Model file for the job. Use its own axes, mm. A direction names the side the tool comes from. Round coordinates to 2 decimals unless told otherwise and drop trailing zeros. Order: outer loops, then holes, each group sorted by start corner. A loop starts at its lowest first (then second) coordinate and runs counter-clockwise, first axis right, second up. Notation, with made-up numbers: (-30, -6) - (-20, -6) arc R18 ccw to (-20, 19) - close; hole circle Ø8 at (-15.5, 43.25). An arc over 180 degrees is marked (long way). Use one line per item in the form item = value.
Autodesk Inventor part; units mm, degrees
ref_plane "Work Plane1" through (-10, 0, 0) normal (1, 0, 0) x (0, 1, 0)
ref_plane "XZ Plane" through (0, 0, 0) normal (0, 1, 0) x (-1, 0, 0)
ref_plane "XY Plane" through (0, 0, 0) normal (0, 0, 1) x (1, 0, 0)
sketch "Sketch1" plane through (0, 0, 0) normal (0, 0, 1) x (1, 0, 0)
  circle A0 centre (0, 0) radius 125
  dimension "d0" = 250
extrude "Extrusion1" add sketch "Sketch1" along normal blind 10
ref_plane "Work Plane1" through (-10, 0, 0) normal (1, 0, 0) x (0, 1, 0)
sketch "Sketch2" plane through (-10, 0, 0) normal (1, 0, 0) x (0, 1, 0)
  line L0 (0, 0) -> (0, 156.8689) construction
  line L1 (125, 10) -> (-125, 10)
  line L2 (0, 10) -> (-87.5, 10)
  line L3 (-87.5, 10) -> (-87.5, 67.2767)
  line L4 (0, 10) -> (66.5, 10)
  line L5 (66.5, 10) -> (66.5, 44.5)
  line L6 (66.5, 44.5) -> (80.6421, 58.6421)
  line L7 (66.5, 44.5) -> (86.5, 44.5) construction
  line L8 (80.6421, 58.6421) -> (-7.7462, 147.0305) construction
  arc A0 (80.6421, 58.6421) -> (-7.7462, 147.0305) centre (36.448, 102.8363) ccw
  line L9 (-7.7462, 147.0305) -> (-87.5, 67.2767)
  line L10 (-7.7462, 147.0305) -> (127.2538, 147.0305) construction
  circle A1 centre (36.448, 102.8363) radius 22.75
  dimension "d4" = 87.5
  dimension "d6" = 66.5
  dimension "d7" = 34.5
  dimension "d8" = 20
  dimension "d9" = 45
  dimension "d10" = 125
  dimension "d11" = 135
  dimension "d12" = 45.5
extrude "Extrusion2" add sketch "Sketch2" against normal blind 55
fillet "Fillet1" radius 100 1 edges at (-37.5, -87.5, 67.2767)
fillet "Fillet2" radius 50 1 edges at (-37.5, 66.5, 44.5)
sketch "Sketch3" plane through (-65, 0, 0) normal (-1, 0, 0) x (0, 0, 1)
  line L0 (25.8553, -87.5) -> (10, -87.5)
  line L1 (10, -87.5) -> (25.8553, -87.5)
  arc A0 (25.8553, -87.5) -> (96.566, -58.2107) centre (25.8553, 12.5) ccw
  arc A1 (25.8553, -87.5) -> (96.566, -58.2107) centre (25.8553, 12.5) ccw
  line L2 (96.566, -58.2107) -> (147.0305, -7.7462)
  line L3 (96.566, -58.2107) -> (147.0305, -7.7462)
  arc A2 (147.0305, -7.7462) -> (58.6421, 80.6421) centre (102.8363, 36.448) ccw
  arc A3 (147.0305, -7.7462) -> (58.9231, 80.9213) centre (102.8363, 36.448) ccw
  arc A4 (23.7925, 66.5) -> (58.9231, 80.9213) centre (23.7925, 116.5) ccw
  arc A5 (23.7925, 66.5) -> (58.9231, 80.9213) centre (23.7925, 116.5) ccw
  line L4 (44.5, 66.5) -> (10, 66.5)
  line L5 (23.7925, 66.5) -> (10, 66.5)
  line L6 (10, 66.5) -> (10, -87.5)
  arc A6 (139.9594, -0.6751) -> (65.9492, 73.8056) centre (102.8363, 36.448) ccw
  line L7 (139.9594, -0.6751) -> (117.7788, -23.5781)
  line L8 (0, 0) -> (182.0155, 0) construction
  line L9 (0, -125) -> (0, 125) construction
  line L10 (10, 0) -> (10, -65) construction
  line L11 (10, -65) -> (20, -65)
  arc A7 (20, -65) -> (117.7788, -23.5781) centre (20, 71.1171) ccw
  line L12 (10, 0) -> (10, 40) construction
  arc A8 (10, 40) -> (65.9492, 73.8056) centre (-32.4537, 173.4637) ccw
  dimension "d16" = 10
  dimension "d17" = 65
  dimension "d18" = 10
  dimension "d19" = 40
extrude "Extrusion3" cut sketch "Sketch3" against normal blind 19.5 contours L6 A8 A6 L7 A7 L11
sketch "Sketch4" plane through (-45.5, 0, 0) normal (-1, 0, 0) x (0, 0, 1)
  line L0 (143.3452, 39.9686) -> (60.7799, -45.2853) construction
  line L1 (139.9594, -0.6751) -> (117.7788, -23.5781) construction
  circle A0 centre (102.8363, 36.448) radius 22.75 construction
  line L2 (102.2737, 74.1744) -> (28.4952, -2.0066) construction
  line L3 (100.9974, 75.3281) -> (145.8599, 31.8805) construction
  line L4 (22.9611, 6.1258) -> (80.8137, -49.9023) construction
  line L5 (140.5203, 37.0517) -> (68.1686, -37.656)
  line L6 (68.1686, -37.656) -> (29.8809, -0.5758)
  line L7 (29.8809, -0.5758) -> (102.2326, 74.1319)
  line L8 (102.2326, 74.1319) -> (140.5203, 37.0517)
  point P0 (0, 0)
  dimension "d24" = 26.65
  dimension "d25" = 26.65
  dimension "d26" = 26.65
  dimension "d27" = 104
extrude "Extrusion4" cut sketch "Sketch4" against normal blind 30.4
sketch "Sketch5" plane through (-45.5, 0, 0) normal (-1, 0, 0) x (0, 0, 1)
  line L0 (147.2746, 42.9) -> (108.2076, 80.7349) construction
  line L1 (102.2326, 74.1319) -> (140.5203, 37.0517) construction
  circle A0 centre (134.4241, 55.3452) radius 3.3
  circle A1 centre (121.0581, 68.2898) radius 3.3
  line L2 (121.3764, 55.5918) -> (127.7411, 61.8175) construction
  line L3 (140.5203, 37.0517) -> (68.1686, -37.656) construction
  line L4 (104.3444, -0.3021) -> (66.0567, 36.7781) construction
  line L5 (29.8809, -0.5758) -> (102.2326, 74.1319) construction
  circle A2 centre (49.6892, -32.149) radius 3.3
  circle A3 centre (36.3231, -19.2044) radius 3.3
  point P0 (0, 0)
  dimension "d30" = 8.9
  dimension "d31" = 6.6
  dimension "d32" = 6.6
  dimension "d33" = 9.3
  dimension "d34" = 9.3
extrude "Extrusion5" cut sketch "Sketch5" against normal blind 19
properties part number "Final Waist"
(1) Slice it at A-A on z = 72.5. Give the cut face in (x, y).
Report:
outline = (-65, -75.95) - (-10, -75.95) - (-10, 91.09) - (-65, 91.09) - (-65, 79.3) - (-45.5, 79.3) - (-45.5, 43.43) - (-15.1, 43.43) - (-15.1, -33.18) - (-45.5, -33.18) - (-45.5, -54.47) - (-65, -54.47) - close
(2) Pull direction Z, two halves, no side cores. Call faces 1 (the face through (-37.885, -80.097, 63.615)), 2 (the face through (-36.133, -31.158, 52.837)), 3 (the face through (-37, -87.5, 18)): released by +Z, released by -Z, zero draft, split by the parting line, or undercut.
Report:
face_1 = released by +Z
face_2 = undercut
face_3 = zero draft
(3) Probe probe 1 along Z at (x, y) = (-19.5, 74); probe 2 along Z at (x, y) = (68, 99); probe 3 along Y at (x, z) = (-27, 110). List the from-to ranges inside material, lowest first. Write a range as [from, to].
Report:
probe_1 = [0, 10], [50.13, 102.1], [102.37, 152.8]
probe_2 = [0, 10]
probe_3 = [-44.78, 5.54], [66.61, 98.54]
(4) Pin check, flat tips, straight feed: pin 1 (5 mm diameter, centred on y = 23, z = 142.5, fed in from +X); pin 2 (12.5 mm diameter, centred on x = -38, z = 20.5, fed in from -Y); pin 3 (2 mm diameter, centred on y = 55.5, z = 134.5, fed in from -X); pin 4 (6 mm diameter, centred on x = -95, y = -87.5, fed in from +Z). Stop position of each tip, or through.
Report:
pin_1 = -10
pin_2 = -87.5
pin_3 = -26.5
pin_4 = through
(5) Slice it at D-D on x = -99.5. Give the cut face in (y, z).
Report:
outline = (-75.66, 0) - (75.66, 0) - (75.66, 10) - (-75.66, 10) - close
(6) Slice it at B-B on x = -34.5. Count the separate pieces of the cut face and the enclosed holes in it, then the cut area to 3 significant figures.
Report:
separate_pieces = 1
enclosed_holes = 5
area = 18,100 mm2
(7) Tool access for faces 4 (the face through (-37, 66.5, 17)), 5 (the face through (-124.88, -5.5, 4.93)), 6 (the face through (-65, -36, 105)), 7 (the face through (-26.5, 68, 121)): list every direction of +Z, -Z, +X, -X, +Y, -Y with a clear straight run to the whole face (end or side of a thin tool).
Report:
face_4 = +X, -X, +Y
face_5 = +Z, -Z
face_6 = +Z, -X, +Y, -Y
face_7 = -X
(8) Slice it at C-C on x = 0. Give the cut face in (y, z).
Report:
outline = (-125, 0) - (125, 0) - (125, 10) - (-125, 10) - close
